from build123d import *

# Parameters (mm, degrees)
SKETCH1_W           = 255
SKETCH1_H           = 130
SKETCH1_R           = 4.05
SKETCH1_R_2         = 4
SKETCH1_R_3         = 3
BOSS_EXTRUDE1_DEPTH = 21
CHAMFER1_SIZE       = 2
CHAMFER5_SIZE       = 1
CHAMFER6_SIZE       = 1


with BuildPart() as part:
    # Sketch1 → Boss-Extrude1 (new body)
    with BuildSketch(Plane(origin=(0, 0, 0), x_dir=(1, 0, 0), z_dir=(0, 1, 0))):
        with Locations((127.5, 65)):
            Rectangle(SKETCH1_W, SKETCH1_H)
        with Locations(Location((73.68, 112.78, 0), (0, 0, 270))):
            Circle(SKETCH1_R, mode=Mode.SUBTRACT)
        with Locations(Location((133.87, 111.67, 0), (0, 0, 270))):
            Circle(SKETCH1_R, mode=Mode.SUBTRACT)
        with Locations(Location((133.61, 31.48, 0), (0, 0, 270))):
            Circle(SKETCH1_R, mode=Mode.SUBTRACT)
        with Locations(Location((74.69, 31.92, 0), (0, 0, 270))):
            Circle(SKETCH1_R, mode=Mode.SUBTRACT)
        with Locations(Location((26.03, 90.25, 0), (0, 0, 270))):
            Circle(SKETCH1_R_2, mode=Mode.SUBTRACT)
        with Locations(Location((26.03, 40.14, 0), (0, 0, 270))):
            Circle(SKETCH1_R_2, mode=Mode.SUBTRACT)
        with Locations(Location((21, 112.78, 0), (0, 0, 270))):
            Circle(SKETCH1_R, mode=Mode.SUBTRACT)
        with Locations(Location((239, 111.67, 0), (0, 0, 270))):
            Circle(SKETCH1_R, mode=Mode.SUBTRACT)
        with Locations(Location((239, 31.48, 0), (0, 0, 270))):
            Circle(SKETCH1_R, mode=Mode.SUBTRACT)
        with Locations(Location((21, 23, 0), (0, 0, 270))):
            Circle(SKETCH1_R, mode=Mode.SUBTRACT)
        with Locations(Location((65, 65, 0), (0, 0, 270))):
            Circle(SKETCH1_R_3, mode=Mode.SUBTRACT)
        with Locations(Location((190, 65, 0), (0, 0, 270))):
            Circle(SKETCH1_R_3, mode=Mode.SUBTRACT)
        with Locations(Location((147, 95, 0), (0, 0, 270))):
            Circle(SKETCH1_R_3, mode=Mode.SUBTRACT)
        with Locations(Location((55, 18, 0), (0, 0, 270))):
            Circle(SKETCH1_R_3, mode=Mode.SUBTRACT)
    extrude(amount=-BOSS_EXTRUDE1_DEPTH)

    # Chamfer1
    chamfer1_edges = [part.edges().sort_by_distance(p)[0] for p in [
        (127.5, 0, -130),
        (255, 0, -65),
        (127.5, 0, 0),
        (0, 0, -65),
    ]]
    chamfer(chamfer1_edges, length=CHAMFER1_SIZE)

    # Chamfer5
    chamfer5_edges = [part.edges().sort_by_distance(p)[0] for p in [
        (65, 0, -68),
        (190, 0, -68),
        (147, 0, -98),
        (55, 0, -21),
    ]]
    chamfer(chamfer5_edges, length=CHAMFER5_SIZE)

    # Chamfer6
    chamfer6_edges = [part.edges().sort_by_distance(p)[0] for p in [
        (26.03, 0, -94.25),
        (26.03, 0, -44.14),
    ]]
    chamfer(chamfer6_edges, length=CHAMFER6_SIZE)


solid = part.part
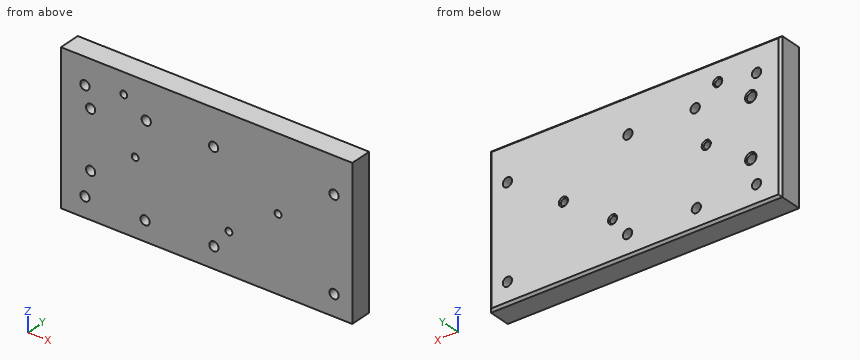
CAD build for the part. Positions are in the model's coordinates, mm. Round coordinates to 2 decimals unless told otherwise and drop trailing zeros. Write each loop counter-clockwise with the first axis right and the second up, starting at its lowest first coordinate (ties: lowest second). Pieces come first, ordered by that corner, then holes.
(1) Slice it at C-C, the plane x = 147. Write the cut outline in (y, z).
(2) Slice it at A-A, the plane z = -65. Write the cut outline in (x, y).
(3) Slice it at B-B, the plane y = -5.75. Count the separate pieces of the cut face and the enclosed holes in it, and give its area (3 significant figures).
(4) Probe line 1 along X through (y, z) = (-8.75, -31.92); line 2 along X through (y, z) = (-8, -31.48); line 3 along X through (y, z) = (-8.5, -65). List the from-to ranges inside material, lowest first.
(5) Slice it at D-D, the plane z = -40.14. Write the cut outline in (x, y), and give its area (3 significant figures).
From the geometry:
1. outline: (-21, -130) - (-2, -130) - (0, -128) - (0, -99) - (-1, -98) - (-21, -98) - close; (-21, -92) - (-1, -92) - (0, -91) - (0, -2) - (-2, 0) - (-21, 0) - close
2. outline: (0, -21) - (62, -21) - (62, -1) - (61, 0) - (2, 0) - (0, -2) - close; (68, -21) - (187, -21) - (187, -1) - (186, 0) - (69, 0) - (68, -1) - close; (193, -21) - (255, -21) - (255, -2) - (253, 0) - (194, 0) - (193, -1) - close
3. separate pieces: 1
3. enclosed holes: 14
3. area: 32,500 mm2
4. line 1: x = 0 to 70.64, 78.74 to 129.58, 137.64 to 234.97, 243.03 to 255
4. line 2: x = 0 to 70.66, 78.72 to 129.56, 137.66 to 234.95, 243.05 to 255
4. line 3: x = 0 to 62, 68 to 187, 193 to 255
5. outline: (0, -21) - (22.03, -21) - (22.03, -1) - (21.03, 0) - (2, 0) - (0, -2) - close; (30.03, -21) - (255, -21) - (255, -2) - (253, 0) - (31.03, 0) - (30.03, -1) - close
5. area: 5,180 mm2
